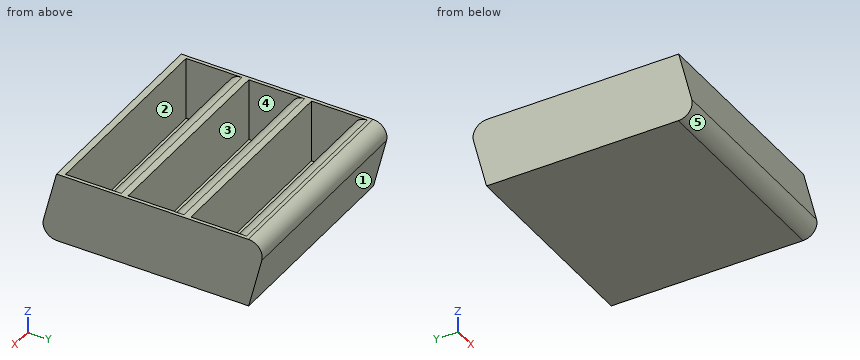
from build123d import *

# Parameters (mm, degrees)
F0_W     = 60.2
F0_H     = 60.2
F2_W     = 60.2
F2_H     = 60.2
F4_W     = 58.2
F4_H     = 12
F5_DEPTH = 18
F6_R     = 4
F7_SIZE  = 3


with BuildPart() as f3:
    # F0 (on Top) → F3 section 0
    with BuildSketch(Plane.XY):
        Rectangle(F0_W, F0_H)
    # F2 (on offset) → F3 section 1
    with BuildSketch(Plane.XY.offset(20)):
        with Locations((0, 5)):
            Rectangle(F2_W, F2_H)
    loft()

    # F4 (on face) → F5 (cut)
    with BuildSketch(Plane.XY.offset(20)):
        with Locations((0, -17.1)):
            Rectangle(F4_W, F4_H)
        with Locations((0, 0.9)):
            Rectangle(F4_W, F4_H)
        with Locations((0, 18.9)):
            Rectangle(F4_W, F4_H)
    extrude(amount=-F5_DEPTH, mode=Mode.SUBTRACT)

    # F6
    f6_edges = [f3.edges().sort_by_distance(p)[0] for p in [
        (0, -30.1, 0),
        (0, 35.1, 20),
        (0, -11.1, 20),
        (0, 6.9, 20),
        (0, 24.9, 20),
    ]]
    fillet(f6_edges, radius=F6_R)

    # F7
    f7_edges = [f3.edges().sort_by_distance(p)[0] for p in [
        (0, 24.9, 2),
        (0, 6.9, 2),
        (0, -11.1, 2),
    ]]
    chamfer(f7_edges, length=F7_SIZE)


solid = f3.part
Verification items for the finished model (mm, model axes). Face numbers are marked on the shaded views. A direction names the side the tool comes from. Give positions to 0.01 mm unless a question says otherwise; leave off trailing zeros. Order: outer loops, then holes, each group sorted by start corner. A loop starts at its lowest first (then second) coordinate and runs counter-clockwise, first axis right, second up. Notation, with made-up numbers: M -16.75,40.25 L -5.75,40.25 A7 cw -5.75,50.25 Z; hole C -12,26.5 d4. An arc over 180 degrees is marked long. Answer as a JSON object with one key per item and string values. Group by question number.
1) Access from +Z, -Z, +X, -X, +Y, -Y to the whole of each face (thin tool, end or side, straight path). Record for the marked faces 1 and 2.
2) Depth check by flat-ended pin: pin 1 Ø5 at (x, y) = (7.5, -12) entering from +Z; pin 2 Ø5.5 at (x, z) = (11, 12.5) entering from -Y; pin 3 Ø8 at (x, z) = (1.5, 11) entering from +Y. Enter the tip coordinate at first touch or a pass-through.
3) Cross-section at A-A (x = -10). Enter the section's corners in (y, z), then the cut area to 3 significant figures.
4) Cross-section at B-B (z = 10.75). Give the number of separate pieces and of enclosed holes in the cut face, then the cut area to 3 significant figures.
5) Mould release check, pull along X, two halves, no side actions. Record for the marked faces 3, 4 and 5: released by +X, released by -X, zero draft, split by the parting line, or undercut.
6) Scan lines: line 1 along X through (y, z) = (-22, 10.25); line 2 along Y through (x, z) = (-23.5, 6.25); line 3 along Y through (x, z) = (-3.5, 11.5) (3 decimals). Record each from-to range of solid material in increasing order. Write a range as [from, to].
Result sheet:
{
 "1": {"face 1": "-Z, +X, -X, +Y", "face 2": "+Z"},
 "2": {"pin 1": "stops at z = 19.2", "pin 2": "stops at y = -27.66", "pin 3": "stops at y = 33.85"},
 "3": {"outline": "M -28.86,4.97 A4 ccw -24.98,0 L 30.1,0 L 33.86,15.03 A4 ccw 29.98,20 L 28.9,20 A4 ccw 24.9,16 L 24.9,5 L 21.9,2 L 12.9,2 L 12.9,20 L 10.9,20 A4 ccw 6.9,16 L 6.9,5 L 3.9,2 L -5.1,2 L -5.1,20 L -7.1,20 A4 ccw -11.1,16 L -11.1,5 L -14.1,2 L -23.1,2 L -23.1,20 L -25.1,20 Z", "area": "547 mm2"},
 "4": {"separate pieces": "1", "enclosed holes": "3", "area": "1,530 mm2"},
 "5": {"face 3": "undercut", "face 4": "undercut", "face 5": "zero draft"},
 "6": {"line 1": "x = [-30.1, -29.1], [29.1, 30.1]", "line 2": "y = [-28.54, -23.1], [-11.1, -5.1], [6.9, 12.9], [24.9, 31.66]", "line 3": "y = [-27.225, -23.1], [-11.1, -5.1], [6.9, 12.9], [24.9, 32.975]"}
}
